```python
from build123d import *

# Parameters (mm, degrees)
ESQUISSE1_W                   = 270
ESQUISSE1_H                   = 213
BOSS_EXTRU_1_DEPTH            = 6
ESQUISSE3_R                   = 9.45
ESQUISSE3_R_2                 = 1.5
ENL_V_MAT_EXTRU_1_DEPTH       = 10
ESQUISSE4_R                   = 3
ENL_V_MAT_EXTRU_2_DEPTH       = 10
ENL_V_MAT_EXTRU_11_DEPTH      = 173.055950202
ENL_V_MAT_EXTRU_11_DEPTH_BACK = 173.055950202
ESQUISSE7_W                   = 6
ESQUISSE7_H                   = 30
ESQUISSE7_H_2                 = 27
ENL_V_MAT_EXTRU_13_DEPTH      = 10
ESQUISSE8_W                   = 40
ESQUISSE8_H                   = 6
BOSS_EXTRU_2_DEPTH            = 6
ENL_V_MAT_EXTRU_14_DEPTH      = 10
ENL_V_MAT_EXTRU_15_DEPTH      = 6
ESQUISSE11_W                  = 6
ESQUISSE11_H                  = 15
ENL_V_MAT_EXTRU_16_DEPTH      = 10
ESQUISSE12_R                  = 1.65
ENL_V_MAT_EXTRU_17_DEPTH      = 176.833017377
ESQUISSE14_W                  = 30
ESQUISSE14_H                  = 6
BOSS_EXTRU_3_DEPTH            = 6
ENL_V_MAT_EXTRU_18_DEPTH      = 176.833017377
ESQUISSE16_R                  = 4
ENL_V_MAT_EXTRU_19_DEPTH      = 1
ESQUISSE17_R                  = 2.995
ENL_V_MAT_EXTRU_20_DEPTH      = 3
ESQUISSE18_R                  = 1.5
ENL_V_MAT_EXTRU_21_DEPTH      = 13


with BuildPart() as part:
    # Esquisse1 → Boss.-Extru.1 (new body)
    with BuildSketch(Plane.XY):
        Rectangle(ESQUISSE1_W, ESQUISSE1_H)
    extrude(amount=BOSS_EXTRU_1_DEPTH)

    # Esquisse3 → Enlèv. mat.-Extru.1 (cut)
    with BuildSketch(Plane.XY.offset(6)):
        with Locations((-100, -21.5)):
            Circle(ESQUISSE3_R)
        with Locations((58.459193141, 0.881055644)):
            Circle(ESQUISSE3_R_2)
        with Locations((49.798939104, 5.881055644)):
            Circle(ESQUISSE3_R_2)
        with Locations((42.298939104, -7.109325413)):
            Circle(ESQUISSE3_R_2)
        with Locations((50.959193141, -12.109325413)):
            Circle(ESQUISSE3_R_2)
        with Locations((70.011752025, -23.109325413)):
            Circle(ESQUISSE3_R_2)
        with Locations((78.672006063, -28.109325413)):
            Circle(ESQUISSE3_R_2)
        with Locations((86.172006063, -15.118944356)):
            Circle(ESQUISSE3_R_2)
        with Locations((77.511752025, -10.118944356)):
            Circle(ESQUISSE3_R_2)
    extrude(amount=-ENL_V_MAT_EXTRU_1_DEPTH, mode=Mode.SUBTRACT)

    # Esquisse4 → Enlèv. mat.-Extru.2 (cut)
    with BuildSketch(Plane.XY.offset(6)):
        with Locations((-105, 82.5)):
            Circle(ESQUISSE4_R)
    extrude(amount=-ENL_V_MAT_EXTRU_2_DEPTH, mode=Mode.SUBTRACT)

    # Esquisse5 → Enlèv. mat.-Extru.11 (cut, two sides: drawn at the far end of the back side and taken through both)
    with BuildSketch(Plane.XY.offset(6).offset(-ENL_V_MAT_EXTRU_11_DEPTH_BACK)):
        Polygon((135, -36.5), (53.963742643, -43.589753853), (-55, -106.5), (135, -106.5), align=None)
    extrude(amount=ENL_V_MAT_EXTRU_11_DEPTH + ENL_V_MAT_EXTRU_11_DEPTH_BACK, mode=Mode.SUBTRACT)

    # Esquisse7 → Enlèv. mat.-Extru.13 (cut)
    with BuildSketch(Plane.XY.offset(6)):
        with Locations((132, 91.5)):
            Rectangle(ESQUISSE7_W, ESQUISSE7_H)
        with Locations((132, -17)):
            Rectangle(ESQUISSE7_W, ESQUISSE7_H_2)
        with Locations((132, 34)):
            Rectangle(ESQUISSE7_W, ESQUISSE7_H_2)
    extrude(amount=-ENL_V_MAT_EXTRU_13_DEPTH, mode=Mode.SUBTRACT)

    # Esquisse8 → Boss.-Extru.2 (add)
    with BuildSketch(Plane(origin=(0, 106.5, 0), x_dir=(1, 0, 0), z_dir=(0, 1, 0))):
        with Locations((85, -3)):
            Rectangle(ESQUISSE8_W, ESQUISSE8_H)
        with Locations((5, -3)):
            Rectangle(ESQUISSE8_W, ESQUISSE8_H)
        with Locations((-75, -3)):
            Rectangle(ESQUISSE8_W, ESQUISSE8_H)
    extrude(amount=BOSS_EXTRU_2_DEPTH)

    # Esquisse9 → Enlèv. mat.-Extru.14 (cut)
    with BuildSketch(Plane(origin=(0, 0, 0), x_dir=(-1, 0, 0), z_dir=(0, 0, -1))):
        Polygon((-110.35, -38.656595556), (-79.413742643, -41.363167367), (-78.890808186, -35.385999178), (-109.827065544, -32.679427367), align=None)
    extrude(amount=-ENL_V_MAT_EXTRU_14_DEPTH, mode=Mode.SUBTRACT)

    # Esquisse10 → Enlèv. mat.-Extru.15 (cut)
    with BuildSketch(Plane(origin=(0, 0, 0), x_dir=(-1, 0, 0), z_dir=(0, 0, -1))):
        Polygon((-32.03555308, -56.25), (-10.384917986, -68.75), (-7.384917986, -63.553847577), (-29.03555308, -51.053847577), align=None)
        Polygon((11.265717109, -81.25), (32.916352203, -93.75), (35.916352203, -88.553847577), (14.265717109, -76.053847577), align=None)
    extrude(amount=-ENL_V_MAT_EXTRU_15_DEPTH, mode=Mode.SUBTRACT)

    # Esquisse11 → Enlèv. mat.-Extru.16 (cut)
    with BuildSketch(Plane(origin=(0, 0, 0), x_dir=(-1, 0, 0), z_dir=(0, 0, -1))):
        with Locations((72, 52)):
            Rectangle(ESQUISSE11_W, ESQUISSE11_H)
        with Locations((72, 83)):
            Rectangle(ESQUISSE11_W, ESQUISSE11_H)
    extrude(amount=-ENL_V_MAT_EXTRU_16_DEPTH, mode=Mode.SUBTRACT)

    # Esquisse12 → Enlèv. mat.-Extru.17 (cut, through all)
    with BuildSketch(Plane.XY.offset(6)):
        with Locations((-25, 52.5)):
            Circle(ESQUISSE12_R)
        with Locations((35, 22.5)):
            Circle(ESQUISSE12_R)
        with Locations((-5, 42.5)):
            Circle(ESQUISSE12_R)
        with Locations((15, 32.5)):
            Circle(ESQUISSE12_R)
        with Locations((55, 12.5)):
            Circle(ESQUISSE12_R)
        with Locations((75, 2.5)):
            Circle(ESQUISSE12_R)
        with Locations((-45, 62.5)):
            Circle(ESQUISSE12_R)
    extrude(amount=-ENL_V_MAT_EXTRU_17_DEPTH, mode=Mode.SUBTRACT)

    # Esquisse14 → Boss.-Extru.3 (add)
    with BuildSketch(Plane.XZ.offset(106.5)):
        with Locations((-95, 3)):
            Rectangle(ESQUISSE14_W, ESQUISSE14_H)
    extrude(amount=BOSS_EXTRU_3_DEPTH)

    # Esquisse15 → Enlèv. mat.-Extru.18 (cut, through all)
    with BuildSketch(Plane.XY.offset(6)):
        Polygon((105, 106.5), (129, 106.5), (129, 76.5), align=None)
    extrude(amount=-ENL_V_MAT_EXTRU_18_DEPTH, mode=Mode.SUBTRACT)

    # Esquisse16 → Enlèv. mat.-Extru.19 (cut)
    with BuildSketch(Plane.XY.offset(6)):
        with Locations((-45, 62.5)):
            Circle(ESQUISSE16_R)
        with Locations((-25, 52.5)):
            Circle(ESQUISSE16_R)
        with Locations((-5, 42.5)):
            Circle(ESQUISSE16_R)
        with Locations((15, 32.5)):
            Circle(ESQUISSE16_R)
        with Locations((35, 22.5)):
            Circle(ESQUISSE16_R)
        with Locations((55, 12.5)):
            Circle(ESQUISSE16_R)
        with Locations((75, 2.5)):
            Circle(ESQUISSE16_R)
    extrude(amount=-ENL_V_MAT_EXTRU_19_DEPTH, mode=Mode.SUBTRACT)

    # Esquisse17 → Enlèv. mat.-Extru.20 (cut)
    with BuildSketch(Plane.XY.offset(6)):
        with Locations((-75, 109.5)):
            Circle(ESQUISSE17_R)
        with Locations((5, 109.5)):
            Circle(ESQUISSE17_R)
        with Locations((85, 109.5)):
            Circle(ESQUISSE17_R)
        with Locations((132, 60)):
            Circle(ESQUISSE17_R)
        with Locations((132, 9)):
            Circle(ESQUISSE17_R)
        with Locations((-1.940399562, -72.401923789)):
            Circle(ESQUISSE17_R)
        with Locations((118.78170639, -34.90745732)):
            Circle(ESQUISSE17_R)
        with Locations((66.699841688, -39.464030057)):
            Circle(ESQUISSE17_R)
        with Locations((-45.241669751, -97.401923789)):
            Circle(ESQUISSE17_R)
    extrude(amount=-ENL_V_MAT_EXTRU_20_DEPTH, mode=Mode.SUBTRACT)

    # Esquisse18 → Enlèv. mat.-Extru.21 (cut)
    with BuildSketch(Plane.XY.offset(6)):
        with Locations((-75, 109.5)):
            Circle(ESQUISSE18_R)
        with Locations((5, 109.5)):
            Circle(ESQUISSE18_R)
        with Locations((85, 109.5)):
            Circle(ESQUISSE18_R)
        with Locations((132, 60)):
            Circle(ESQUISSE18_R)
        with Locations((132, 9)):
            Circle(ESQUISSE18_R)
        with Locations((118.78170639, -34.90745732)):
            Circle(ESQUISSE18_R)
        with Locations((66.699841688, -39.464030057)):
            Circle(ESQUISSE18_R)
        with Locations((-1.940399562, -72.401923789)):
            Circle(ESQUISSE18_R)
        with Locations((-45.241669751, -97.401923789)):
            Circle(ESQUISSE18_R)
    extrude(amount=-ENL_V_MAT_EXTRU_21_DEPTH, mode=Mode.SUBTRACT)


solid = part.part
```
CAD build for the part. Positions are in the model's coordinates, mm. A direction names the side the tool comes from. Round coordinates to 2 decimals unless told otherwise and drop trailing zeros. Loops run counter-clockwise (first coordinate to the right, second up) from the corner with the lowest first, then second, coordinate; pieces in that order, holes last. Notation, with made-up numbers: M 54.5,26.5 L 81.5,26.5 A21 ccw 81.5,40.5 Z; hole C -16.5,36.25 d4. An arc over 180 degrees is marked long. Return JSON: item names as keys, results as strings. Group by question number.
(1) Tool access for faces 1 (the flat face through (25, 109, 3)), 2 (the cylindrical face through (-5.521, 46.466, 5.507)), 3 (the flat face through (-75, 83, 3)), 4 (the flat face through (132, 47.5, 3)): list every direction of +Z, -Z, +X, -X, +Y, -Y with a clear straight run to the whole face (end or side of a thin tool).
(2) Wall check: probe 1 along X at (y, z) = (32, 5.5); probe 2 along X at (y, z) = (-22.5, 5.25); probe 3 along Y at (x, z) = (132, 5.1) (3 decimals). Give the ranges that are in metal, low to high. Write a range as [from, to].
(3) Saw through at A-A, the plane x = 22. List the corners of the cut face in (y, z).
(4) Drop flat-ended pins along their axis: P1, Ø3, axis at y = 81, z = 4, coming from the +X side; P2, Ø6.5, axis at x = -45.5, y = -96, coming from the +Z side; P3, Ø1.8, axis at x = 78.67, y = -28.11, coming from the +Z side; P4, Ø3.5, axis at x = 132, y = 60, coming from the +Z side. Give the stop position or say it passes through.
(5) Mould opens along Y. For faces 5 (the flat face through (-75, 112.5, 2)), 6 (the cylindrical face through (-91.27, -25.12, 3.04)), 7 (the flat face through (-15, 109, 3)) say: +Y half, -Y half, draft (parallel to the pull), parting line (faces both ways), or undercut.
Answer list:
{
 "1": {"face 1": "+Z, -Z, +Y", "face 2": "+Z", "face 3": "+Z, -Z", "face 4": "+Z, -Z, +X"},
 "2": {"probe 1": "[-135, 11.03], [18.97, 129]", "probe 2": "[-135, -109.4], [-90.6, 68.64], [71.38, 129]", "probe 3": "[-36.762, -30.5], [-3.5, 6.005], [11.995, 20.5], [47.5, 57.005], [62.995, 76.5]"},
 "3": {"outline": "M -55.12,0 L 112.5,0 L 112.5,6 L -55.12,6 Z"},
 "4": {"P1": "x = 126.6", "P2": "z = 6", "P3": "through", "P4": "z = 3"},
 "5": {"face 5": "+Y half", "face 6": "undercut", "face 7": "draft"}
}
